```python
from build123d import *

# Parameters (mm, degrees)
SKETCH_1_W          = 32.5
SKETCH_1_H          = 26.5
SKETCH_2_R          = 23
CUT_EXTRUDE_1_DEPTH = 15
SKETCH_3_R          = 8
EXTRUDE_1_DEPTH     = 4
CUT_EXTRUDE_2_DEPTH = 12.5


with BuildPart() as part:
    # 草图1 → 旋转1 (revolve)
    with BuildSketch(Plane.XY):
        with Locations((16.25, 13.25)):
            Rectangle(SKETCH_1_W, SKETCH_1_H)
    revolve(axis=Axis((0, 54.381188119, 0), (0, -1, 0)))

    # 草图2 → 切除-拉伸1 (cut)
    with BuildSketch(Plane(origin=(0, 26.5, 0), x_dir=(1, 0, 0), z_dir=(0, 1, 0))):
        Circle(SKETCH_2_R)
    extrude(amount=-CUT_EXTRUDE_1_DEPTH, mode=Mode.SUBTRACT)

    # 草图3 → 凸台-拉伸1 (add)
    with BuildSketch(Plane(origin=(0, 11.5, 0), x_dir=(1, 0, 0), z_dir=(0, 1, 0))):
        Circle(SKETCH_3_R)
        Polygon((-3.5, 6.062177826), (3.5, 6.062177826), (7, 0), (3.5, -6.062177826), (-3.5, -6.062177826), (-7, 0), align=None, mode=Mode.SUBTRACT)
    extrude(amount=EXTRUDE_1_DEPTH)

    # 草图4 → 切除-拉伸2 (cut, through all)
    with BuildSketch(Plane(origin=(0, 11.5, 0), x_dir=(1, 0, 0), z_dir=(0, 1, 0))):
        with BuildLine():
            Line((-0.925251662, 7.9463142), (-2.807719573, 22.827980874))
            ThreePointArc((-2.807719573, 22.827980874), (0, 23), (2.807719573, 22.827980874))
            Line((2.807719573, 22.827980874), (0.925251662, 7.9463142))
            ThreePointArc((0.925251662, 7.9463142), (0, 8), (-0.925251662, 7.9463142))
        make_face()
        with BuildLine():
            Line((5.816576204, 5.492489532), (16.824381237, 15.682480544))
            ThreePointArc((16.824381237, 15.682480544), (14.784115023, 17.619022192), (12.522705284, 19.292015249))
            Line((12.522705284, 19.292015249), (4.399008416, 6.68197014))
            ThreePointArc((4.399008416, 6.68197014), (5.142300877, 6.128355545), (5.816576204, 5.492489532))
        make_face()
        with BuildLine():
            Line((7.986260097, 0.46866797), (22.968727938, 1.198973275))
            ThreePointArc((22.968727938, 1.198973275), (22.650578319, 3.993908086), (21.993617163, 6.729101282))
            Line((21.993617163, 6.729101282), (7.664923567, 2.29105799))
            ThreePointArc((7.664923567, 2.29105799), (7.878462024, 1.389185421), (7.986260097, 0.46866797))
        make_face()
        with BuildLine():
            Line((6.419084133, -4.774448544), (18.365751568, -13.845546914))
            ThreePointArc((18.365751568, -13.845546914), (19.918584287, -11.5), (21.173471141, -8.98243396))
            Line((21.173471141, -8.98243396), (7.344335794, -3.171865656))
            ThreePointArc((7.344335794, -3.171865656), (6.92820323, -4), (6.419084133, -4.774448544))
        make_face()
        with BuildLine():
            Line((1.848347363, -7.783547522), (5.169235927, -22.411581826))
            ThreePointArc((5.169235927, -22.411581826), (7.866463296, -21.612930278), (10.446022654, -20.490988524))
            Line((10.446022654, -20.490988524), (3.58725168, -7.15063811))
            ThreePointArc((3.58725168, -7.15063811), (2.736161147, -7.517540966), (1.848347363, -7.783547522))
        make_face()
        with BuildLine():
            Line((-3.58725168, -7.15063811), (-10.446022654, -20.490988524))
            ThreePointArc((-10.446022654, -20.490988524), (-7.866463296, -21.612930278), (-5.169235927, -22.411581826))
            Line((-5.169235927, -22.411581826), (-1.848347363, -7.783547522))
            ThreePointArc((-1.848347363, -7.783547522), (-2.736161147, -7.517540966), (-3.58725168, -7.15063811))
        make_face()
        with BuildLine():
            Line((-7.344335794, -3.171865656), (-21.173471141, -8.98243396))
            ThreePointArc((-21.173471141, -8.98243396), (-19.918584287, -11.5), (-18.365751568, -13.845546914))
            Line((-18.365751568, -13.845546914), (-6.419084133, -4.774448544))
            ThreePointArc((-6.419084133, -4.774448544), (-6.92820323, -4), (-7.344335794, -3.171865656))
        make_face()
        with BuildLine():
            Line((-7.664923567, 2.29105799), (-21.993617163, 6.729101282))
            ThreePointArc((-21.993617163, 6.729101282), (-22.650578319, 3.993908086), (-22.968727938, 1.198973275))
            Line((-22.968727938, 1.198973275), (-7.986260097, 0.46866797))
            ThreePointArc((-7.986260097, 0.46866797), (-7.878462024, 1.389185421), (-7.664923567, 2.29105799))
        make_face()
        with BuildLine():
            Line((-4.399008416, 6.68197014), (-12.522705284, 19.292015249))
            ThreePointArc((-12.522705284, 19.292015249), (-14.784115023, 17.619022192), (-16.824381237, 15.682480544))
            Line((-16.824381237, 15.682480544), (-5.816576204, 5.492489532))
            ThreePointArc((-5.816576204, 5.492489532), (-5.142300877, 6.128355545), (-4.399008416, 6.68197014))
        make_face()
    extrude(amount=-CUT_EXTRUDE_2_DEPTH, mode=Mode.SUBTRACT)


solid = part.part
```
Can you work these out from the model? Positions are in its coordinate system, mm. A direction names the side the tool comes from. Coordinates: 2 decimals unless noted, no trailing zeros. Loops run counter-clockwise (first coordinate to the right, second up) from the corner with the lowest first, then second, coordinate; pieces in that order, holes last. Notation, with made-up numbers: M 57,66 L 94,66 A20 cw 94,88 Z; hole C 20,14.25 d3. An arc over 180 degrees is marked long. Put each result on its own line as item: value. Start each with the question number.
(1) I need wall thicknesses on probe 1 along X at (y, z) = (3.5, -16.5); probe 2 along Z at (x, y) = (0, 16.5); probe 3 along Z at (x, y) = (-18, 5). Which ranges of each line are inside material? Lowest first, please.
(2) Imagine slicing it at B-B on z = -21.5. List the corners of the cut face in (x, y) for me, and give its area (3 significant figures).
(3) Imagine slicing it at D-D on x = 11.5. List the corners of the cut face in (y, z) for me.
(4) Which directions (+Z, -Z, +X, -X, +Y, -Y) give clear straight access to the entire face, cutting with the end or side of a thin tool? Please do faces 1 (the face through (-14.73, 5.83, -4.48)), 2 (the face through (0, 0, 0)), 3 (the face through (-17, 11.5, 3)).
(5) Will these pins go through, and if not, where does the flat tip stop? pin 1 Ø6 at (x, z) = (-4, -12.5) entering from +Y; pin 2 Ø12 at (y, z) = (20, -14.5) entering from -X; pin 3 Ø3 at (x, y) = (-0.5, 14) entering from -Z; pin 4 Ø2 at (x, z) = (-22.5, -25) entering from +Y.
(6) Imagine slicing it at C-C on y = 18. List the corners of the cut face in (x, z) for me, and give its area (3 significant figures).
(7) We'd pull the mould along Z, two halves only. Please class faces 4 (the face through (31, 13.44, 9.76)), 5 (the face through (1.88, 5.83, -15.49)), 6 (the face through (8, 26.5, 22)): +Z half, -Z half, draft (parallel to the pull), parting line (faces both ways), or undercut.
(8) Imagine slicing it at A-A on x = 0. List the corners of the cut face in (y, z) for me, and give its area (4 significant figures).
Worked answers:
1. probe 1: x = -28 to -16.02, -10.72 to -2.01, 2.01 to 10.72, 16.02 to 28
1. probe 2: z = -32.5 to -23, 23 to 32.5
1. probe 3: z = -27.06 to -5.49, -0.96 to 7.65, 13.57 to 27.06
2. outline: M -24.37,0 L -2.64,0 L -2.64,11.5 L -8.17,11.5 L -8.17,26.5 L -24.37,26.5 Z; M 2.64,0 L 24.37,0 L 24.37,26.5 L 8.17,26.5 L 8.17,11.5 L 2.64,11.5 Z
2. area: 986 mm2
3. outline: M 0,-30.4 L 26.5,-30.4 L 26.5,-19.92 L 11.5,-19.92 L 11.5,-17.7 L 0,-17.7 Z; M 0,-10.75 L 11.5,-10.75 L 11.5,-3.48 L 0,-3.48 Z; M 0,-0.64 L 11.5,-0.64 L 11.5,4.92 L 0,4.92 Z; M 0,8.63 L 11.5,8.63 L 11.5,19.92 L 26.5,19.92 L 26.5,30.4 L 0,30.4 Z
4. face 1: +Y, -Y
4. face 2: +Z, -Z, +X, -X, -Y
4. face 3: +Y
5. pin 1: stops at y = 11.5
5. pin 2: stops at x = -31.37
5. pin 3: stops at z = -32.5
5. pin 4: passes through
6. outline: C 0,0 d65; hole C 0,0 d46
6. area: 1,660 mm2
7. face 4: parting line
7. face 5: undercut
7. face 6: draft
8. outline: M 0,-32.5 L 26.5,-32.5 L 26.5,-23 L 0,-23 Z; M 0,-8 L 15.5,-8 L 15.5,-6.06 L 11.5,-6.06 L 11.5,6.06 L 15.5,6.06 L 15.5,8 L 11.5,8 L 11.5,23 L 26.5,23 L 26.5,32.5 L 0,32.5 Z
8. area: 875.5 mm2
